from build123d import *

# Parameters (mm, degrees)
SKETCH1_W                    = 723.9
SKETCH1_H                    = 200.152
BASE_FLANGE1_DEPTH           = 1.6002
EDGE_FLANGE1_STRIP_W         = 7.874
EDGE_FLANGE1_STRIP_H         = 1.6002
EDGE_FLANGE1_STRIP_CUT_DEPTH = 723.9
EDGE_FLANGE1_DEPTH           = 723.9
EDGE_FLANGE2_STRIP_W         = 7.874
EDGE_FLANGE2_STRIP_H         = 1.6002
EDGE_FLANGE2_STRIP_CUT_DEPTH = 723.9
EDGE_FLANGE2_DEPTH           = 723.9
SKETCH12_R                   = 3.175
SKETCH12_R_2                 = 14.2875
CUT_EXTRUDE1_DEPTH           = 376.744991019
SKETCH13_R                   = 3.175
CUT_EXTRUDE2_DEPTH           = 395.072064437
EDGE_FLANGE3_DEPTH           = 195.4784
EDGE_FLANGE3_BEND_DEPTH      = 195.4784
SKETCH20_R                   = 3.175
CUT_EXTRUDE3_DEPTH           = 736.498403773
SKETCH22_R                   = 5.55625
SKETCH22_R_2                 = 2.5527
SKETCH22_R_3                 = 2.0447
SKETCH22_R_4                 = 11.10615
CUT_EXTRUDE4_DEPTH           = 378.946139007
SKETCH23_R                   = 3.175
CUT_EXTRUDE5_DEPTH           = 378.996519072


# Sheet-metal steps are written as plain solids
with BuildPart() as part:
    # Base-Flange1: sheet metal written as solids
    # Sketch1 → Base-Flange1 (new body)
    with BuildSketch(Plane.XY):
        Rectangle(SKETCH1_W, SKETCH1_H)
    extrude(amount=-BASE_FLANGE1_DEPTH)

    # Edge-Flange1: sheet metal written as solids
    # Edge-Flange1 strip (on a plane across the edge) → Edge-Flange1 strip cut (cut)
    with BuildSketch(Plane(origin=(361.95, 100.076, 0), x_dir=(0, -1, 0), z_dir=(-1, 0, 0))):
        with Locations((-1.6002, -0.8001)):
            Rectangle(EDGE_FLANGE1_STRIP_W, EDGE_FLANGE1_STRIP_H)
    extrude(amount=EDGE_FLANGE1_STRIP_CUT_DEPTH, mode=Mode.SUBTRACT)

    # Edge-Flange1 section (on a plane across the edge) → Edge-Flange1 (add)
    with BuildSketch(Plane(origin=(361.95, 100.076, 0), x_dir=(0, -1, 0), z_dir=(-1, 0, 0))):
        with BuildLine():
            Line((0, 0.7366), (0, 11.0998))
            Line((0, 11.0998), (1.6002, 11.0998))
            Line((1.6002, 11.0998), (1.6002, 0.7366))
            ThreePointArc((1.6002, 0.7366), (1.815945145, 0.215745145), (2.3368, 0))
            Line((2.3368, 0), (2.3368, -1.6002))
            ThreePointArc((2.3368, -1.6002), (0.684432874, -0.915767126), (0, 0.7366))
        make_face()
    extrude(amount=EDGE_FLANGE1_DEPTH)

    # Edge-Flange2: sheet metal written as solids
    # Edge-Flange2 strip (on a plane across the edge) → Edge-Flange2 strip cut (cut)
    with BuildSketch(Plane(origin=(-361.95, -100.076, 0), x_dir=(0, 1, 0), z_dir=(1, 0, 0))):
        with Locations((-1.6002, -0.8001)):
            Rectangle(EDGE_FLANGE2_STRIP_W, EDGE_FLANGE2_STRIP_H)
    extrude(amount=EDGE_FLANGE2_STRIP_CUT_DEPTH, mode=Mode.SUBTRACT)

    # Edge-Flange2 section (on a plane across the edge) → Edge-Flange2 (add)
    with BuildSketch(Plane(origin=(-361.95, -100.076, 0), x_dir=(0, 1, 0), z_dir=(1, 0, 0))):
        with BuildLine():
            Line((0, 0.7366), (0, 11.0998))
            Line((0, 11.0998), (1.6002, 11.0998))
            Line((1.6002, 11.0998), (1.6002, 0.7366))
            ThreePointArc((1.6002, 0.7366), (1.815945145, 0.215745145), (2.3368, 0))
            Line((2.3368, 0), (2.3368, -1.6002))
            ThreePointArc((2.3368, -1.6002), (0.684432874, -0.915767126), (0, 0.7366))
        make_face()
    extrude(amount=EDGE_FLANGE2_DEPTH)

    # Sketch12 → Cut-Extrude1 (cut, through all)
    with BuildSketch(Plane(origin=(0, 0, -1.6002), x_dir=(-1, 0, 0), z_dir=(0, 0, -1))):
        with Locations((-207.518, -14.351)):
            Circle(SKETCH12_R)
        with Locations((0, -17.526)):
            Circle(SKETCH12_R)
        with Locations((207.518, -14.351)):
            Circle(SKETCH12_R)
        with Locations((-320.548, 23.268449438)):
            Circle(SKETCH12_R_2)
    extrude(amount=-CUT_EXTRUDE1_DEPTH, mode=Mode.SUBTRACT)

    # Sketch13 → Cut-Extrude2 (cut, through all)
    with BuildSketch(Plane(origin=(0, 0, -108.356399896), x_dir=(-1, 0, 0), z_dir=(0, 0, -1))):
        with Locations(Location((-309.118, -65.151, 0), (0, 0, 90))):
            Circle(SKETCH13_R)
        with Locations(Location((-104.638118017, -65.151, 0), (0, 0, 90))):
            Circle(SKETCH13_R)
        with Locations(Location((-104.638118017, 49.149, 0), (0, 0, 90))):
            Circle(SKETCH13_R)
        with Locations(Location((104.638118017, 49.149, 0), (0, 0, 90))):
            Circle(SKETCH13_R)
        with Locations(Location((104.638118017, -65.151, 0), (0, 0, 90))):
            Circle(SKETCH13_R)
        with Locations(Location((309.118, -65.151, 0), (0, 0, 90))):
            Circle(SKETCH13_R)
        with Locations(Location((309.118, 49.149, 0), (0, 0, 90))):
            Circle(SKETCH13_R)
    extrude(amount=-CUT_EXTRUDE2_DEPTH, mode=Mode.SUBTRACT)

    # Edge-Flange3: sheet metal written as solids
    # Edge-Flange3 section (on a plane across the edge) → Edge-Flange3 (add)
    with BuildSketch(Plane(origin=(-362.6866, 97.7392, 0), x_dir=(1, 0, 0), z_dir=(0, -1, 0))):
        with BuildLine():
            Line((-1.6002, 0.7366), (-1.6002, 11.0998))
            Line((-1.6002, 11.0998), (0, 11.0998))
            Line((0, 11.0998), (0, 0.7366))
            ThreePointArc((0, 0.7366), (0.215745145, 0.215745145), (0.7366, 0))
            Line((0.7366, 0), (0.7366, -1.6002))
            ThreePointArc((0.7366, -1.6002), (-0.915767126, -0.915767126), (-1.6002, 0.7366))
        make_face()
    extrude(amount=EDGE_FLANGE3_DEPTH)

    # Edge-Flange3 section 2 (on a plane across the edge) → Edge-Flange3 bend (add)
    with BuildSketch(Plane(origin=(362.6866, -97.7392, 0), x_dir=(-1, 0, 0), z_dir=(0, 1, 0))):
        with BuildLine():
            Line((-1.6002, 0.7366), (-1.6002, 11.0998))
            Line((-1.6002, 11.0998), (0, 11.0998))
            Line((0, 11.0998), (0, 0.7366))
            ThreePointArc((0, 0.7366), (0.215745145, 0.215745145), (0.7366, 0))
            Line((0.7366, 0), (0.7366, -1.6002))
            ThreePointArc((0.7366, -1.6002), (-0.915767126, -0.915767126), (-1.6002, 0.7366))
        make_face()
    extrude(amount=EDGE_FLANGE3_BEND_DEPTH)

    # Sketch20 → Cut-Extrude3 (cut, through all)
    with BuildSketch(Plane.ZY.offset(364.2868)):
        with Locations((5.9182, 72.3392)):
            Circle(SKETCH20_R)
        with Locations((5.9182, 0)):
            Circle(SKETCH20_R)
        with Locations((5.9182, -72.3392)):
            Circle(SKETCH20_R)
    extrude(amount=-CUT_EXTRUDE3_DEPTH, mode=Mode.SUBTRACT)

    # Sketch22 → Cut-Extrude4 (cut, through all)
    with BuildSketch(Plane.XY):
        with Locations((266.978063087, -15.466550562)):
            Circle(SKETCH22_R)
        with Locations((249.960063087, -8.481550562)):
            Circle(SKETCH22_R_2)
        with Locations((249.960063087, -14.323550562)):
            Circle(SKETCH22_R_3)
        with Locations((249.960063087, 55.018449438)):
            Circle(SKETCH22_R_2)
        with Locations((249.960063087, 60.860449438)):
            Circle(SKETCH22_R_3)
        with Locations((266.978063087, 62.003449438)):
            Circle(SKETCH22_R)
        with Locations((292.378063087, 62.003449438)):
            Circle(SKETCH22_R)
        with Locations((317.778063087, 62.003449438)):
            Circle(SKETCH22_R)
        with Locations((338.860063087, 62.003449438)):
            Circle(SKETCH22_R_2)
        with Locations((338.860063087, 67.845449438)):
            Circle(SKETCH22_R_3)
        with Locations((338.860063087, -15.466550562)):
            Circle(SKETCH22_R_2)
        with Locations((338.860063087, -21.308550562)):
            Circle(SKETCH22_R_3)
        with Locations((279.8318, 23.268449438)):
            Circle(SKETCH22_R_4)
        with Locations((292.378063087, -15.466550562)):
            Circle(SKETCH22_R)
        with Locations((317.778063087, -15.466550562)):
            Circle(SKETCH22_R)
    extrude(amount=-CUT_EXTRUDE4_DEPTH, mode=Mode.SUBTRACT)

    # Sketch23 → Cut-Extrude5 (cut, through all)
    with BuildSketch(Plane(origin=(0, 0, -1.6002), x_dir=(-1, 0, 0), z_dir=(0, 0, -1))):
        with Locations((-349.25, 85.0392)):
            Circle(SKETCH23_R)
    extrude(amount=-CUT_EXTRUDE5_DEPTH, mode=Mode.SUBTRACT)


solid = part.part
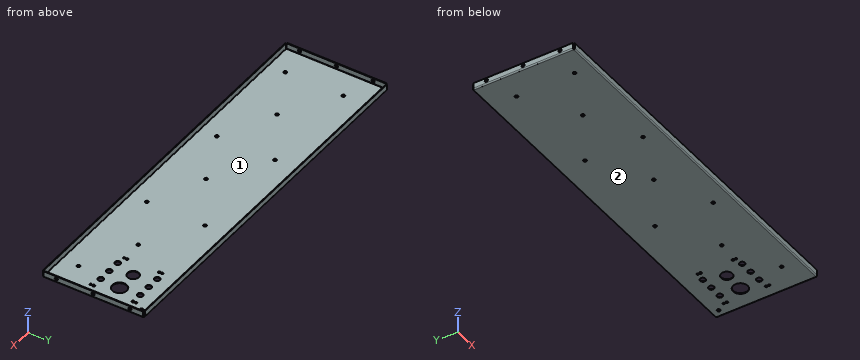
Design review of the part built by this model. Coordinates are the model's own, in mm. Face numbers are marked on the shaded views. Give positions to 0.01 mm unless a question says otherwise; leave off trailing zeros. Write each loop counter-clockwise with the first axis right and the second up, starting at its lowest first coordinate (ties: lowest second). Pieces come first, ordered by that corner, then holes. Notation, with made-up numbers: M 2,52.25 L 39,52.25 A26 ccw 39,81.25 Z; hole C -3,-7 d9. An arc over 180 degrees is marked long. Return JSON: item names as keys, results as strings. Group by question number.
Item 1: Clearance check with flat-ended pins moving along their axes: pin 1 Ø0.7 at (y, z) = (-99, 6) entering from -X; pin 2 Ø5.5 at (x, y) = (249.96, -14.32) entering from +Z; pin 3 Ø1.9 at (x, z) = (363, 2) entering from +Y. State where each tip first meets the part, or that it passes through.
Item 2: Wall thickness on line 1 along Y through (x, z) = (-224.5, 5.5); line 2 along X through (y, z) = (74, 1); line 3 along Y through (x, z) = (327, 0.5): over which ranges is each line inside the solid? List them lowest first.
Item 3: The part is to be moulded in two halves that separate along Y. For the marked faces 1 and 2, say which applies: pulls with the +Y half, pulls with the -Y half, needs draft (parallel to the pull), parting line crosses it, or undercut.
Item 4: Take a section at A-A (x = 13). Give the boundary of the cut face in (y, z).
Return value:
{
 "1": {"pin 1": "stops at x = -361.95", "pin 2": "stops at z = 0", "pin 3": "stops at y = 97.74"},
 "2": {"line 1": "y = -100.08 to -98.48, 98.48 to 100.08", "line 2": "x = -364.29 to -362.69, 362.69 to 364.29", "line 3": "y = -100.06 to -98.44, 98.44 to 100.06"},
 "3": {"face 1": "undercut", "face 2": "needs draft"},
 "4": {"outline": "M -100.08,0.74 A2.34 ccw -97.74,-1.6 L 97.74,-1.6 A2.34 ccw 100.08,0.74 L 100.08,11.1 L 98.48,11.1 L 98.48,0.74 A0.74 cw 97.74,0 L -97.74,0 A0.74 cw -98.48,0.74 L -98.48,11.1 L -100.08,11.1 Z"}
}
